Can you work these out from the model? Positions are in its coordinate system, mm. A direction names the side the tool comes from. Give positions to 0.01 mm unless a question says otherwise; leave off trailing zeros. Loops run counter-clockwise (first coordinate to the right, second up) from the corner with the lowest first, then second, coordinate; pieces in that order, holes last. Notation, with made-up numbers: (40, 72.5) - (48, 72.5) arc R28 ccw to (48, 106.5) - close; hole circle Ø10 at (63, 34.25). An arc over 180 degrees is marked (long way). Answer as a JSON object with one key per item and string values. Group by question number.
Item 1: Please list where these lines run through material, in increasing order: L1, parallel to Y at x = 2, z = 1; L2, parallel to X at y = 170, z = -0.65; L3, parallel to Y at x = 73.5, z = -0.2.
Item 2: Suppose I cut it at B-B on z = -0.65. Count the separate pieces of the cut face and the enclosed holes in it, and give its area (3 significant figures).
Item 3: Will these pins go through, and if not, where does the flat tip stop? pin 1 (1 mm diameter, centred on y = 74, z = 0.5, fed in from -X); pin 2 (1.5 mm diameter, centred on x = 86.5, z = -0.5, fed in from -Y); pin 3 (1.5 mm diameter, centred on y = 73.5, z = 0, fed in from +X); pin 4 (8 mm diameter, centred on x = 0, y = 0, fed in from -Z).
Item 4: Thinking about a two-plate mould opening in Y: for faces 1 (the cylindrical face through (-159.42, 120.77, 0.02)), 2 (the cylindrical face through (159.42, -120.77, 0.02)), 3 (the flat face through (13.4, -184.2, 0)), which applies, pulls with the +Y half, pulls with the -Y half, needs draft (parallel to the pull), parting line crosses it, or undercut?
Item 5: Suppose I cut it at A-A on x = 117.5. Write out the boundary of the cut face in (y, z).
Item 6: Suppose I cut it at C-C on y = -56.5. Write out the boundary of the cut face in (x, z), and give its area (3 significant figures).
Item 7: Which directions (+Z, -Z, +X, -X, +Y, -Y) give clear straight access to the entire face, cutting with the end or side of a thin tool? Please do faces 4 (the cylindrical face through (-77.671, 184.302, 0.018)), 5 (the flat face through (184.2, 13.4, 0)).
from build123d import *

# Parameters (mm, degrees)
F0_R          = 5.05
F1_DEPTH      = 1.25
F1_DEPTH_BACK = 1.25


with BuildPart() as f1:
    # F0 (on Top) → F1 (new body, two sides)
    with BuildSketch(Plane.XY) as f1_sk:
        with BuildLine():
            Line((-169.263686, -0.654074), (-197.850831, -29.241219))
            ThreePointArc((-197.850831, -29.241219), (-184.022709, -78.330343), (-158.228698, -122.326118))
            Line((-158.228698, -122.326118), (-157.736526, -122.041962))
            Line((-157.736526, -122.041962), (-147.7568, -84.797118))
            ThreePointArc((-147.7568, -84.797118), (-147.792977, -84.522325), (-147.573088, -84.691052))
            Line((-147.573088, -84.691052), (-146.365681, -85.014576))
            ThreePointArc((-146.365681, -85.014576), (-146.090888, -84.978399), (-146.259615, -85.198287))
            Line((-146.259615, -85.198287), (-156.723236, -124.249053))
            ThreePointArc((-156.723236, -124.249053), (-120.203169, -159.847422), (-75.867013, -185.051875))
            Line((-75.867013, -185.051875), (-75.582858, -184.559702))
            Line((-75.582858, -184.559702), (-85.562583, -147.314858))
            ThreePointArc((-85.562583, -147.314858), (-85.73131, -147.094969), (-85.456517, -147.131146))
            Line((-85.456517, -147.131146), (-84.24911, -146.807623))
            ThreePointArc((-84.24911, -146.807623), (-84.029221, -146.638896), (-84.065398, -146.913689))
            Line((-84.065398, -146.913689), (-73.601777, -185.964455))
            ThreePointArc((-73.601777, -185.964455), (-24.175287, -198.533512), (26.823176, -198.193131))
            Line((26.823176, -198.193131), (26.823176, -197.624819))
            Line((26.823176, -197.624819), (-0.441942, -170.359701))
            ThreePointArc((-0.441942, -170.359701), (-0.698008, -170.253635), (-0.441942, -170.147569))
            Line((-0.441942, -170.147569), (0.441942, -169.263686))
            ThreePointArc((0.441942, -169.263686), (0.548008, -169.00762), (0.654074, -169.263686))
            Line((0.654074, -169.263686), (29.241219, -197.850831))
            ThreePointArc((29.241219, -197.850831), (78.330343, -184.022709), (122.326118, -158.228698))
            Line((122.326118, -158.228698), (122.041962, -157.736526))
            Line((122.041962, -157.736526), (84.797118, -147.7568))
            ThreePointArc((84.797118, -147.7568), (84.522325, -147.792977), (84.691052, -147.573088))
            Line((84.691052, -147.573088), (85.014576, -146.365681))
            ThreePointArc((85.014576, -146.365681), (84.978399, -146.090888), (85.198287, -146.259615))
            Line((85.198287, -146.259615), (124.249053, -156.723236))
            ThreePointArc((124.249053, -156.723236), (159.847422, -120.203169), (185.051875, -75.867013))
            Line((185.051875, -75.867013), (184.559702, -75.582858))
            Line((184.559702, -75.582858), (147.314858, -85.562583))
            ThreePointArc((147.314858, -85.562583), (147.094969, -85.73131), (147.131146, -85.456517))
            Line((147.131146, -85.456517), (146.807623, -84.24911))
            ThreePointArc((146.807623, -84.24911), (146.638896, -84.029221), (146.913689, -84.065398))
            Line((146.913689, -84.065398), (185.964455, -73.601777))
            ThreePointArc((185.964455, -73.601777), (198.533512, -24.175287), (198.193131, 26.823176))
            Line((198.193131, 26.823176), (197.624819, 26.823176))
            Line((197.624819, 26.823176), (170.359701, -0.441942))
            ThreePointArc((170.359701, -0.441942), (170.253635, -0.698008), (170.147569, -0.441942))
            Line((170.147569, -0.441942), (169.263686, 0.441942))
            ThreePointArc((169.263686, 0.441942), (169.00762, 0.548008), (169.263686, 0.654074))
            Line((169.263686, 0.654074), (197.850831, 29.241219))
            ThreePointArc((197.850831, 29.241219), (184.022709, 78.330343), (158.228698, 122.326118))
            Line((158.228698, 122.326118), (157.736526, 122.041962))
            Line((157.736526, 122.041962), (147.7568, 84.797118))
            ThreePointArc((147.7568, 84.797118), (147.792977, 84.522325), (147.573088, 84.691052))
            Line((147.573088, 84.691052), (146.365681, 85.014576))
            ThreePointArc((146.365681, 85.014576), (146.090888, 84.978399), (146.259615, 85.198287))
            Line((146.259615, 85.198287), (156.723236, 124.249053))
            ThreePointArc((156.723236, 124.249053), (120.203169, 159.847422), (75.867013, 185.051875))
            Line((75.867013, 185.051875), (75.582858, 184.559702))
            Line((75.582858, 184.559702), (85.562583, 147.314858))
            ThreePointArc((85.562583, 147.314858), (85.73131, 147.094969), (85.456517, 147.131146))
            Line((85.456517, 147.131146), (84.24911, 146.807623))
            ThreePointArc((84.24911, 146.807623), (84.029221, 146.638896), (84.065398, 146.913689))
            Line((84.065398, 146.913689), (73.601777, 185.964455))
            ThreePointArc((73.601777, 185.964455), (24.175287, 198.533512), (-26.823176, 198.193131))
            Line((-26.823176, 198.193131), (-26.823176, 197.624819))
            Line((-26.823176, 197.624819), (0.441942, 170.359701))
            ThreePointArc((0.441942, 170.359701), (0.698008, 170.253635), (0.441942, 170.147569))
            Line((0.441942, 170.147569), (-0.441942, 169.263686))
            ThreePointArc((-0.441942, 169.263686), (-0.548008, 169.00762), (-0.654074, 169.263686))
            Line((-0.654074, 169.263686), (-29.241219, 197.850831))
            ThreePointArc((-29.241219, 197.850831), (-78.330343, 184.022709), (-122.326118, 158.228698))
            Line((-122.326118, 158.228698), (-122.041962, 157.736526))
            Line((-122.041962, 157.736526), (-84.797118, 147.7568))
            ThreePointArc((-84.797118, 147.7568), (-84.522325, 147.792977), (-84.691052, 147.573088))
            Line((-84.691052, 147.573088), (-85.014576, 146.365681))
            ThreePointArc((-85.014576, 146.365681), (-84.978399, 146.090888), (-85.198287, 146.259615))
            Line((-85.198287, 146.259615), (-124.249053, 156.723236))
            ThreePointArc((-124.249053, 156.723236), (-159.847422, 120.203169), (-185.051875, 75.867013))
            Line((-185.051875, 75.867013), (-184.559702, 75.582858))
            Line((-184.559702, 75.582858), (-147.314858, 85.562583))
            ThreePointArc((-147.314858, 85.562583), (-147.094969, 85.73131), (-147.131146, 85.456517))
            Line((-147.131146, 85.456517), (-146.807623, 84.24911))
            ThreePointArc((-146.807623, 84.24911), (-146.638896, 84.029221), (-146.913689, 84.065398))
            Line((-146.913689, 84.065398), (-185.964455, 73.601777))
            ThreePointArc((-185.964455, 73.601777), (-198.533512, 24.175287), (-198.193131, -26.823176))
            Line((-198.193131, -26.823176), (-197.624819, -26.823176))
            Line((-197.624819, -26.823176), (-170.359701, 0.441942))
            ThreePointArc((-170.359701, 0.441942), (-170.253635, 0.698008), (-170.147569, 0.441942))
            Line((-170.147569, 0.441942), (-169.263686, -0.441942))
            ThreePointArc((-169.263686, -0.441942), (-169.00762, -0.548008), (-169.263686, -0.654074))
        make_face()
        Polygon((-5.99273, -161.556222), (-8.149406, -163.712898), (-11.68494, -160.177364), (-9.528264, -158.020688), align=None, mode=Mode.SUBTRACT)
        Polygon((-85.967967, -136.915427), (-88.914041, -137.704825), (-90.208136, -132.875196), (-87.262063, -132.085798), align=None, mode=Mode.SUBTRACT)
        Polygon((-142.908157, -75.588255), (-145.854231, -74.798856), (-144.560136, -69.969227), (-141.614062, -70.758625), align=None, mode=Mode.SUBTRACT)
        Polygon((75.588255, -142.908157), (74.798856, -145.854231), (69.969227, -144.560136), (70.758625, -141.614062), align=None, mode=Mode.SUBTRACT)
        Circle(F0_R, mode=Mode.SUBTRACT)
        Polygon((136.915427, -85.967967), (137.704825, -88.914041), (132.875196, -90.208136), (132.085798, -87.262063), align=None, mode=Mode.SUBTRACT)
        Polygon((161.556222, -5.99273), (163.712898, -8.149406), (160.177364, -11.68494), (158.020688, -9.528264), align=None, mode=Mode.SUBTRACT)
        Polygon((-161.556222, 5.99273), (-163.712898, 8.149406), (-160.177364, 11.68494), (-158.020688, 9.528264), align=None, mode=Mode.SUBTRACT)
        Polygon((-136.915427, 85.967967), (-137.704825, 88.914041), (-132.875196, 90.208136), (-132.085798, 87.262063), align=None, mode=Mode.SUBTRACT)
        Polygon((-75.588255, 142.908157), (-74.798856, 145.854231), (-69.969227, 144.560136), (-70.758625, 141.614062), align=None, mode=Mode.SUBTRACT)
        Polygon((142.908157, 75.588255), (145.854231, 74.798856), (144.560136, 69.969227), (141.614062, 70.758625), align=None, mode=Mode.SUBTRACT)
        Polygon((85.967967, 136.915427), (88.914041, 137.704825), (90.208136, 132.875196), (87.262063, 132.085798), align=None, mode=Mode.SUBTRACT)
        Polygon((5.99273, 161.556222), (8.149406, 163.712898), (11.68494, 160.177364), (9.528264, 158.020688), align=None, mode=Mode.SUBTRACT)
    extrude(amount=F1_DEPTH)
    extrude(f1_sk.sketch, amount=-F1_DEPTH_BACK)


solid = f1.part
Worked out:
{
 "1": {"L1": "y = -199.99 to -172.8, -170.61 to -4.64, 4.64 to 199.99", "L2": "x = -105.36 to -1.39, 0.29 to 77.88, 79.48 to 105.36", "L3": "y = -186 to -145.51, -142.35 to 186"},
 "2": {"separate pieces": "1", "enclosed holes": "13", "area": "125,000 mm2"},
 "3": {"pin 1": "stops at x = -186", "pin 2": "stops at y = -180.68", "pin 3": "stops at x = 186.3", "pin 4": "passes through"},
 "4": {"face 1": "pulls with the +Y half", "face 2": "pulls with the -Y half", "face 3": "undercut"},
 "5": {"outline": "(-161.84, -1.25) - (-156.52, -1.25) - (-156.52, 1.25) - (-161.84, 1.25) - close; (-154.91, -1.25) - (161.84, -1.25) - (161.84, 1.25) - (-154.91, 1.25) - close"},
 "6": {"outline": "(-191.85, -1.25) - (191.85, -1.25) - (191.85, 1.25) - (-191.85, 1.25) - close", "area": "959 mm2"},
 "7": {"face 4": "+Z, -Z, -X, +Y", "face 5": "+Z, -Z"}
}
